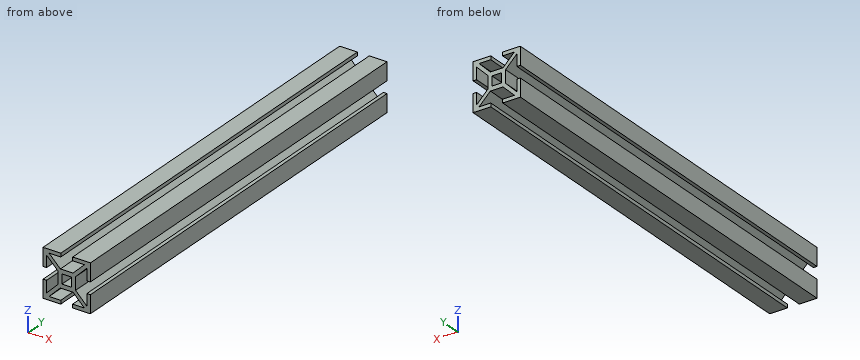
from build123d import *

# Parameters (mm, degrees)
F0_W     = 8
F0_H     = 8
F1_DEPTH = 180


with BuildPart() as f1:
    # F0 (on Front) → F1 (new body, symmetric)
    with BuildSketch(Plane.XZ):
        Polygon((-5, 17), (-5, 20), (-20, 20), (-20, 5), (-17, 5), (-17, 14.87868), (-17, 17), (-14.87868, 17), align=None)
        Polygon((-17, -5), (-20, -5), (-20, -20), (-5, -20), (-5, -17), (-14.87868, -17), (-17, -17), (-17, -14.87868), align=None)
        Polygon((20, -20), (20, -5), (17, -5), (17, -14.87868), (17, -17), (14.87868, -17), (5, -17), (5, -20), align=None)
        Polygon((20, 5), (20, 20), (5, 20), (5, 17), (14.87868, 17), (17, 17), (17, 14.87868), (17, 5), align=None)
        Polygon((17, 17), (14.87868, 17), (5.37868, 7.5), (7.5, 7.5), (7.5, 5.37868), (17, 14.87868), align=None)
        Polygon((-5.37868, 7.5), (-14.87868, 17), (-17, 17), (-17, 14.87868), (-7.5, 5.37868), (-7.5, 7.5), align=None)
        Polygon((-7.5, -5.37868), (-17, -14.87868), (-17, -17), (-14.87868, -17), (-5.37868, -7.5), (-7.5, -7.5), align=None)
        Polygon((17, -17), (17, -14.87868), (7.5, -5.37868), (7.5, -7.5), (5.37868, -7.5), (14.87868, -17), align=None)
        Polygon((7.5, 7.5), (5.37868, 7.5), (-5.37868, 7.5), (-7.5, 7.5), (-7.5, 5.37868), (-7.5, -5.37868), (-7.5, -7.5), (-5.37868, -7.5), (5.37868, -7.5), (7.5, -7.5), (7.5, -5.37868), (7.5, 5.37868), align=None)
        Rectangle(F0_W, F0_H, mode=Mode.SUBTRACT)
    extrude(amount=F1_DEPTH, both=True)


solid = f1.part
Build history of the part. All positions in model axes, mm. Coordinates: 2 decimals unless noted, no trailing zeros. Order: outer loops, then holes, each group sorted by start corner. A loop starts at its lowest first (then second) coordinate and runs counter-clockwise, first axis right, second up. Notation, with made-up numbers: (-2.75, -1) - (47.25, -1) arc R24 ccw to (47.25, 25) - close; hole circle Ø6 at (43.5, -33.75). An arc over 180 degrees is marked (long way). Write item = value, one per line. Start each with the question number.
1) Saw through at A-A on x = 1. Write the cut outline in (y, z), then the cut area to 3 significant figures.
2) Flat gauge pins, fed straight in: pin 1 Ø5.5 at (y, z) = (-45, 1.5) entering from +X; pin 2 Ø9 at (x, y) = (0, -20) entering from +Z. Where does each tip first touch, or does it go through?
3) Wall check: line 1 along X through (y, z) = (-101.5, -9); line 2 along Z through (x, y) = (18, -139.5); line 3 along Z through (x, y) = (-11, 96). Give the ranges that are in metal, low to high. Write a range as from..to.
From the geometry:
q1.outline = (-180, -7.5) - (180, -7.5) - (180, -4) - (-180, -4) - close; (-180, 4) - (180, 4) - (180, 7.5) - (-180, 7.5) - close
q1.area = 2,520 mm^2
q2.pin_1 = 7.5
q2.pin_2 = 7.5
q3.line_1 = -20..-17, -11.12..-6.88, 6.88..11.12, 17..20
q3.line_2 = -20..-5, 5..20
q3.line_3 = -20..-17, -13.12..-8.88, 8.88..13.12, 17..20
